Geometry: final body of the model. Coordinates: model frame, mm. Face numbers are marked on the shaded views. Give positions to 0.01 mm unless a question says otherwise; leave off trailing zeros. Write each loop counter-clockwise with the first axis right and the second up, starting at its lowest first coordinate (ties: lowest second). Pieces come first, ordered by that corner, then holes. Notation, with made-up numbers: (73.5, 29.25) - (130.5, 29.25) arc R12 ccw to (130.5, 39.25) - close; hole circle Ø6 at (65.5, 46). An arc over 180 degrees is marked (long way). Return JSON: item names as keys, results as strings.
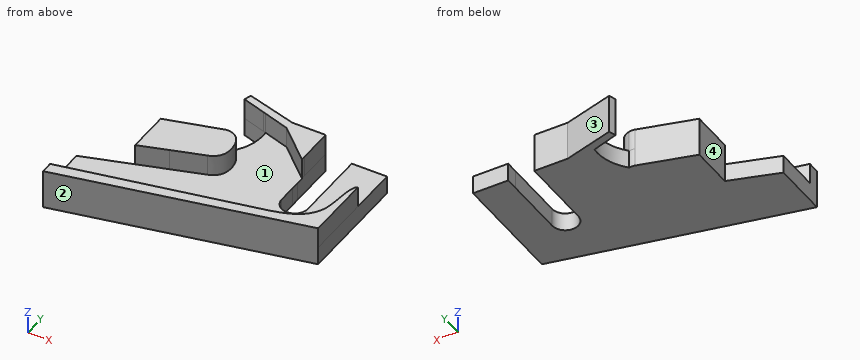
from build123d import *

# Parameters (mm, degrees)
BOSS_EXTRUDE1_DEPTH = 7
BOSS_EXTRUDE3_DEPTH = 15


# Read off the part's stored shape, not the designer's step: Boss-Extrude1
with BuildPart() as part:
    # Boss-Extrude1 outline → Boss-Extrude1 (new body)
    with BuildSketch(Plane.XY):
        with BuildLine():
            add(Edge.make_bspline(
                [(83.179707937, 167.890249892), (88.68617922, 173.842337038), (88.076413708, 182.068482243)],
                knots=[0, 0, 0, 1, 1, 1], degree=2))
            add(Edge.make_bspline(
                [(83.179707937, 167.890249892), (82.472579462, 168.045621317), (81.739782997, 168.056822807), (81.038915385, 167.890249892)],
                knots=[0.899910496, 0.899910496, 0.899910496, 0.899910496, 1, 1, 1, 1], degree=3))
            Line((81.038915385, 167.890249892), (59.792534645, 162.03653789))
            Line((59.792534645, 162.03653789), (59.792534645, 145.583851284))
            Line((59.792534645, 145.583851284), (40.895456025, 139.599456998))
            Line((40.895456025, 139.599456998), (40.895456025, 118.042870489))
            Line((40.895456025, 118.042870489), (134.396295865, 138.100245442))
            Line((134.396295865, 138.100245442), (134.393693517, 182.387043765))
            Line((134.393693517, 182.387043765), (120.894388682, 182.386250529))
            Line((120.894388682, 182.386250529), (120.894655408, 177.847108131))
            Line((120.894655408, 177.847108131), (120.895456025, 177.847108131))
            Line((120.895456025, 177.847108131), (120.895456025, 154.100245399))
            ThreePointArc((120.895456025, 154.100245399), (115.9356337, 149.100406826), (110.896101724, 154.019892645))
            Line((110.896101724, 154.019892645), (110.896055334, 154.022832661))
            ThreePointArc((110.896055334, 154.022832661), (110.895605855, 154.06153787), (110.895456025, 154.100245399))
            Line((110.895456025, 154.100245399), (110.895456025, 161.015247015))
            ThreePointArc((110.895456025, 161.015247015), (110.895045928, 161.07928452), (110.895456025, 161.143322025))
            Line((110.895456025, 161.143322025), (110.895456025, 164.221886849))
            Line((110.895456025, 164.221886849), (110.894388699, 182.385662916))
            Line((110.894388699, 182.385662916), (98.145136748, 182.384913754))
            Line((98.145136748, 182.384913754), (78.980988049, 187.822713754))
            Line((78.980988049, 187.822713754), (78.151089215, 185.147538204))
            Line((78.151089215, 185.147538204), (88.076413708, 182.068482243))
        make_face()
    extrude(amount=BOSS_EXTRUDE1_DEPTH)

    # Sketch2<5> → Boss-Extrude3 (add)
    with BuildSketch(Plane.XY):
        Polygon((87.058497999, 182.38426229), (98.145136748, 182.384913754), (78.980988049, 187.822713754), (78.151089215, 185.147538204), align=None)
        Polygon((97.8963446, 179.022069051), (110.895286898, 167.10010673), (110.895184282, 168.846419808), (110.894388699, 182.385662916), (98.145136748, 182.384913754), (87.058497999, 182.38426229), (88.076413708, 182.068482243), align=None)
        with BuildLine():
            add(Edge.make_bspline(
                [(83.134894854, 152.985445474), (84.153265888, 153.250657791), (85.549452344, 153.989195137), (87.192525807, 155.758725734), (88.24110083, 158.391839128), (88.095392567, 162.20289978), (86.73683171, 166.246070864), (84.288905188, 167.646535258), (83.179707937, 167.890249892)],
                knots=[0, 0, 0, 0, 0.147705893, 0.214614821, 0.335693148, 0.532502628, 0.742910733, 0.899910496, 0.899910496, 0.899910496, 0.899910496], degree=3))
            add(Edge.make_bspline(
                [(83.179707937, 167.890249892), (82.472579462, 168.045621317), (81.739782997, 168.056822807), (81.038915385, 167.890249892)],
                knots=[0.899910496, 0.899910496, 0.899910496, 0.899910496, 1, 1, 1, 1], degree=3))
            Line((81.038915385, 167.890249892), (59.792534645, 162.03653789))
            Line((59.792534645, 162.03653789), (59.792534645, 145.583851284))
            Line((59.792534645, 145.583851284), (70.8963446, 149.100245442))
            Line((70.8963446, 149.100245442), (83.134894854, 152.985445474))
        make_face()
        with BuildLine():
            Line((134.396295865, 138.100245442), (134.394792427, 163.685781747))
            add(Edge.make_bspline(
                [(133.42138155, 162.598444875), (133.72729857, 163.386688135), (134.394792427, 163.685781747)],
                knots=[0, 0, 0, 0.668506509, 0.668506509, 0.668506509], degree=2))
            add(Edge.make_bspline(
                [(115.8963446, 138.100245442), (119.177270844, 138.889647711), (125.41355503, 140.587971019), (133.049150273, 149.2867081), (131.448441996, 157.912006128), (133.42138155, 162.598444875)],
                knots=[0, 0, 0, 0, 0.334742766, 0.521400868, 1, 1, 1, 1], degree=3))
            Line((115.8963446, 138.100245442), (40.895456025, 122.599456998))
            Line((40.895456025, 122.599456998), (40.895456025, 118.042870489))
            Line((40.895456025, 118.042870489), (134.396295865, 138.100245442))
        make_face()
    extrude(amount=BOSS_EXTRUDE3_DEPTH)


solid = part.part
Q1. Section query B-B, the plane z = 12.5. Count the separate pieces of the cut face and the enclosed holes in it, plus the area to 3 significant figures.
Answer key:
{"separate pieces": "3", "enclosed holes": "0", "area": "1,090 mm^2"}
Q2. Section query A-A, the plane x = 94.5. Return the cut outline in (y, z).
Answer key:
{"outline": "(129.54, 0) - (183.42, 0) - (183.42, 15) - (180.08, 15) - (180.08, 7) - (133.68, 7) - (133.68, 15) - (129.54, 15) - close"}
Q3. Pin query (flat end, axial travel): P1, Ø2, axis at x = 74, z = 6.5, coming from the +Y side; P2, Ø4, axis at x = 90.5, z = 11.5, coming from the +Y side; P3, Ø4, axis at y = 178, z = 10, coming from the +X side. Return the tip coordinate at first contact, or that it passes through.
Answer key:
{"P1": "stops at y = 166.23", "P2": "stops at y = 185.12", "P3": "stops at x = 110.89"}
Q4. Section query D-D, the plane x = 108.5. Return the cut outline in (y, z), plus the area to 3 significant figures.
Answer key:
{"outline": "(132.55, 0) - (182.39, 0) - (182.39, 15) - (169.3, 15) - (169.3, 7) - (136.57, 7) - (136.57, 15) - (132.55, 15) - close", "area": "486 mm^2"}
Q5. Mould query, pull axis Y, two halves, no side actions, for the marked faces 1, 2, 3 and 4. Classes: pulls with the +Y half, pulls with the -Y half, needs draft (parallel to the pull), parting line crosses it, or undercut.
Answer key:
{"face 1": "undercut", "face 2": "pulls with the -Y half", "face 3": "pulls with the +Y half", "face 4": "needs draft"}
Q6. Material intervals for probe 1 along Y at (x, z) = (81.5, 9.25); probe 2 along Z at (x, y) = (121, 166.5); probe 3 along X at (y, z) = (174.5, 2), sorted ascending. Write a range as [from, to].
Answer key:
{"probe 1": "y = [126.75, 130.99], [152.47, 167.97], [184.11, 187.11]", "probe 2": "z = [0, 7]", "probe 3": "x = [87.19, 110.89], [120.9, 134.39]"}
Q7. Section query C-C, the plane y = 126. Return the cut outline in (x, z), plus the area to 3 significant figures.
Answer key:
{"outline": "(40.9, 0) - (77.99, 0) - (77.99, 15) - (57.35, 15) - (57.35, 7) - (40.9, 7) - close", "area": "425 mm^2"}
